Study the drawing (mm; zero at the part's minimum x, y, z) and answer. Coordinates: 2 decimals unless noted, no trailing zeros. Write each loop counter-clockwise with the first axis right and the second up, starting at its lowest first coordinate (ties: lowest second). Pieces come first, ordered by that corner, then holes. Notation, with made-up numbers: (87, -26) -> (102, -26) arc R18 ccw to (102, -7) -> close; hole circle Ø8 at (-12.75, 72). An arc over 180 degrees is marked (long way). Answer in a Markdown table with one row per item. Add a question column.
Item 1: Section C-C on z = 3.3 is taken. Write down the section's boundary in (x, y).
Item 2: For a pull along X with two mould halves and no side action, classify the marked faces 1, 2, 3 and 4 as +X half, -X half, draft (parallel to the pull), parting line (faces both ways), or undercut.
Item 3: Straight lines are drawn through the part: line 1 (Y direction, x = 12.5, z = 2.3); line 2 (X direction, y = 19.5, z = 0.2); line 3 (X direction, y = 10.25, z = 1.25). For each, find the intervals that lie inside material, in ascending order. Write a range as from..to.
Item 4: Section D-D on y = 4 is taken. Write down the section's boundary in (x, z), then the cut area to 3 significant figures.
Item 5: Section A-A on y = 12.5 is taken. Write down the section's boundary in (x, z).
Item 6: Given pin 1 Ø2 at (y, z) = (9, 1) entering from -X, flat-ended and moving along its own axis, determine where the tip first touches the part or whether it passes through.
Item 7: Section B-B on x = 12.5 is taken. Write down the section's boundary in (y, z).
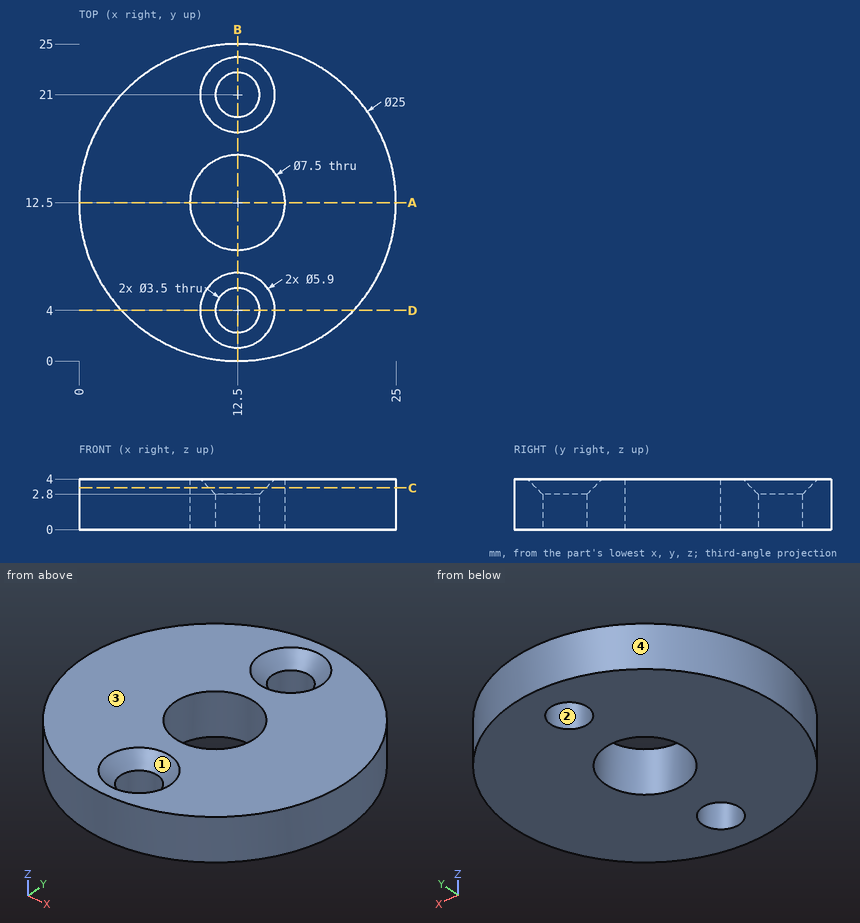
Results below:
| question | item | result |
|---|---|---|
| 1 | outline | circle Ø25 at (12.5, 12.5); hole circle Ø7.5 at (12.5, 12.5); hole circle Ø4.5 at (12.5, 4); hole circle Ø4.5 at (12.5, 21) |
| 2 | face 1 | undercut |
| 2 | face 2 | undercut |
| 2 | face 3 | draft |
| 2 | face 4 | parting line |
| 3 | line 1 | y = 0..2.25, 5.75..8.75, 16.25..19.25, 22.75..25 |
| 3 | line 2 | x = 2.14..11.6, 13.4..22.86 |
| 3 | line 3 | x = 0.2..9.5, 15.5..24.8 |
| 4 | outline | (3.33, 0) -> (10.75, 0) -> (10.75, 2.8) -> (9.55, 4) -> (3.33, 4) -> close; (14.25, 0) -> (21.67, 0) -> (21.67, 4) -> (15.45, 4) -> (14.25, 2.8) -> close |
| 4 | area | 57.9 mm2 |
| 5 | outline | (0, 0) -> (8.75, 0) -> (8.75, 4) -> (0, 4) -> close; (16.25, 0) -> (25, 0) -> (25, 4) -> (16.25, 4) -> close |
| 6 | pin 1 | stops at x = 0.25 |
| 7 | outline | (0, 0) -> (2.25, 0) -> (2.25, 2.8) -> (1.05, 4) -> (0, 4) -> close; (5.75, 0) -> (8.75, 0) -> (8.75, 4) -> (6.95, 4) -> (5.75, 2.8) -> close; (16.25, 0) -> (19.25, 0) -> (19.25, 2.8) -> (18.05, 4) -> (16.25, 4) -> close; (22.75, 0) -> (25, 0) -> (25, 4) -> (23.95, 4) -> (22.75, 2.8) -> close |
